Geometry: final body of the model. Coordinates: model frame, mm. A direction names the side the tool comes from. Coordinates: 2 decimals unless noted, no trailing zeros. Order: outer loops, then holes, each group sorted by start corner. A loop starts at its lowest first (then second) coordinate and runs counter-clockwise, first axis right, second up. Notation, with made-up numbers: (59.5, -27) - (67.5, -27) arc R20 ccw to (67.5, -18) - close; hole circle Ø10 at (83.25, -17). An arc over 180 degrees is marked (long way). Use a Markdown table: item, result. Add a question column.
```python
from build123d import *

# Parameters (mm, degrees)
SKETCH_1_R                   = 1.25
SKETCH_1_R_2                 = 1
EXTRUDE_1_DEPTH              = 5
SKETCH_3_W                   = 35
SKETCH_3_H                   = 7.5
EXTRUDE_2_DEPTH              = 12.5
SKETCH_5_R                   = 2.25
CUT_EXTRUDE_1_DEPTH          = 7.5
FILLET_2_R                   = 40
HOLE_WIZARD_M3_1_D           = 3.2
HOLE_WIZARD_M3_1_CBORE_D     = 6
HOLE_WIZARD_M3_1_CBORE_DEPTH = 3.4
CUT_EXTRUDE_2_DEPTH          = 48.681233206
FILLET_1_R                   = 2


with BuildPart() as part:
    # 草图1 → 凸台-拉伸1 (new body)
    # profile 1 of 2: a face of its own
    with BuildSketch(Plane.XY):
        with BuildLine():
            ThreePointArc((12.5, 18.708286934), (0, 22.5), (-12.5, 18.708286934))
            ThreePointArc((-12.5, 18.708286934), (-22.487606156, -0.746705683), (-11.231408892, -19.496293348))
            Line((-11.231408892, -19.496293348), (-5.24132415, -9.098270229))
            ThreePointArc((-5.24132415, -9.098270229), (-5.254336134, 9.090761892), (10.5, 0))
            ThreePointArc((10.5, 0), (9.090761892, -5.254336134), (5.24132415, -9.098270229))
            Line((5.24132415, -9.098270229), (11.231408892, -19.496293348))
            ThreePointArc((11.231408892, -19.496293348), (19.480204055, -11.259291717), (22.5, 0))
            ThreePointArc((22.5, 0), (19.843134833, 10.606601718), (12.5, 18.708286934))
        make_face()
        with Locations((-13.611805538, -13.611805538)):
            Circle(SKETCH_1_R, mode=Mode.SUBTRACT)
        with Locations((-10.25, -8)):
            Circle(SKETCH_1_R_2, mode=Mode.SUBTRACT)
        with Locations((10.25, -8)):
            Circle(SKETCH_1_R_2, mode=Mode.SUBTRACT)
        with Locations((13.611805538, -13.611805538)):
            Circle(SKETCH_1_R, mode=Mode.SUBTRACT)
        with Locations((-13.611805538, 13.611805538)):
            Circle(SKETCH_1_R, mode=Mode.SUBTRACT)
        with Locations((-10.25, 8)):
            Circle(SKETCH_1_R_2, mode=Mode.SUBTRACT)
        with Locations((10.25, 8)):
            Circle(SKETCH_1_R_2, mode=Mode.SUBTRACT)
        with Locations((13.611805538, 13.611805538)):
            Circle(SKETCH_1_R, mode=Mode.SUBTRACT)
    # profile 2 of 2: a face of its own
    with BuildSketch(Plane.XY):
        with BuildLine():
            Line((-12.5, 37.5), (-12.5, 18.708286934))
            ThreePointArc((-12.5, 18.708286934), (0, 22.5), (12.5, 18.708286934))
            Line((12.5, 18.708286934), (12.5, 37.5))
            Line((12.5, 37.5), (-12.5, 37.5))
        make_face()
    extrude(amount=EXTRUDE_1_DEPTH)

    # 草图3 → 凸台-拉伸2 (add, symmetric)
    with BuildSketch(Plane(origin=(0, 0, 0), x_dir=(0, 0, -1), z_dir=(1, 0, 0))):
        with Locations((-3.5, 33.75)):
            Rectangle(SKETCH_3_W, SKETCH_3_H)
    extrude(amount=EXTRUDE_2_DEPTH, both=True)

    # 草图5 → 切除-拉伸1 (cut, symmetric)
    with BuildSketch(Plane.XZ.offset(-30)):
        with Locations(Location((0, 3.5, 0), (0, 0, 270))):
            Circle(SKETCH_5_R)
    extrude(amount=CUT_EXTRUDE_1_DEPTH, both=True, mode=Mode.SUBTRACT)

    # 圆角2
    # the kernel refuses this fillet: 40 mm, written as the material it adds along each edge
    with BuildSketch(Plane(origin=(-12.5, 18.708286934, -38.008407454), x_dir=(-0.7015991579933682, -0.7125718360298817, 0), z_dir=(0, 0, 1))) as fillet_2_piece_1_section:
        with BuildLine():
            CenterArc((17.230478046, -39.169540108), FILLET_2_R, 101.695565513, 32.859880379)
            Line((-10.833488274, -10.666666667), (0, 0))
            ThreePointArc((0, 0), (4.561008895, -0.467133689), (9.122017789, 0))
        make_face()
    fillet_2_piece_1 = extrude(amount=43.008407454, mode=Mode.PRIVATE)
    fillet_2_piece_1 = split(fillet_2_piece_1, bisect_by=Plane(origin=(-12.133812824, 31.883513777, 0), z_dir=(0, 0, -1)), keep=Keep.TOP, mode=Mode.PRIVATE)
    fillet_2_piece_1 = split(fillet_2_piece_1, bisect_by=Plane(origin=(-12.133812824, 30, -7), z_dir=(0, 1, 0)), keep=Keep.TOP, mode=Mode.PRIVATE)
    fillet_2_piece_1 = split(fillet_2_piece_1, bisect_by=Plane(origin=(-12.133812824, 31.883513777, -14), z_dir=(0, 0, 1)), keep=Keep.TOP, mode=Mode.PRIVATE)
    add(fillet_2_piece_1)
    with BuildSketch(Plane(origin=(-12.5, 18.708286934, 0), x_dir=(-0.7015991579933694, -0.7125718360298806, 0), z_dir=(0, 0, 1))) as fillet_2_piece_2_section:
        with BuildLine():
            CenterArc((17.230478046, -39.169540108), FILLET_2_R, 101.695565513, 32.859880379)
            Line((-10.833488274, -10.666666667), (0, 0))
            ThreePointArc((0, 0), (4.561008895, -0.467133689), (9.122017789, 0))
        make_face()
    fillet_2_piece_2 = extrude(amount=5, mode=Mode.PRIVATE)
    fillet_2_piece_2 = split(fillet_2_piece_2, bisect_by=Plane(origin=(-13.82835822, 30, 2.5), z_dir=(0, -1, 0)), keep=Keep.TOP, mode=Mode.PRIVATE)
    add(fillet_2_piece_2)
    with BuildSketch(Plane(origin=(-12.5, 18.708286934, 0), x_dir=(-0.7015991579933694, -0.7125718360298806, 0), z_dir=(0, 0, 1))) as fillet_2_piece_3_section:
        with BuildLine():
            CenterArc((17.230478046, -39.169540108), FILLET_2_R, 101.695565513, 32.859880379)
            Line((-10.833488274, -10.666666667), (0, 0))
            ThreePointArc((0, 0), (4.561008895, -0.467133689), (9.122017789, 0))
        make_face()
    fillet_2_piece_3 = extrude(amount=5, mode=Mode.PRIVATE)
    fillet_2_piece_3 = split(fillet_2_piece_3, bisect_by=Plane(origin=(-12.133812824, 30, 2.5), z_dir=(0, 1, 0)), keep=Keep.TOP, mode=Mode.PRIVATE)
    add(fillet_2_piece_3)
    with BuildSketch(Plane(origin=(-12.5, 18.708286934, 0), x_dir=(-0.7015991579933694, -0.7125718360298806, 0), z_dir=(0, 0, 1))) as fillet_2_piece_4_section:
        with BuildLine():
            CenterArc((17.230478046, -39.169540108), FILLET_2_R, 101.695565513, 32.859880379)
            Line((-10.833488274, -10.666666667), (0, 0))
            ThreePointArc((0, 0), (4.561008895, -0.467133689), (9.122017789, 0))
        make_face()
    fillet_2_piece_4 = extrude(amount=43.008407454, mode=Mode.PRIVATE)
    fillet_2_piece_4 = split(fillet_2_piece_4, bisect_by=Plane(origin=(-12.133812824, 31.883513777, 5), z_dir=(0, 0, 1)), keep=Keep.TOP, mode=Mode.PRIVATE)
    fillet_2_piece_4 = split(fillet_2_piece_4, bisect_by=Plane(origin=(-12.133812824, 30, 13), z_dir=(0, 1, 0)), keep=Keep.TOP, mode=Mode.PRIVATE)
    fillet_2_piece_4 = split(fillet_2_piece_4, bisect_by=Plane(origin=(-12.133812824, 31.883513777, 21), z_dir=(0, 0, -1)), keep=Keep.TOP, mode=Mode.PRIVATE)
    add(fillet_2_piece_4)
    with BuildSketch(Plane(origin=(12.5, 18.708286934, -38.008407454), x_dir=(0.7015991579933666, -0.7125718360298834, 0), z_dir=(0, 0, 1))) as fillet_2_piece_5_section:
        with BuildLine():
            CenterArc((17.230478046, 39.169540108), FILLET_2_R, 225.444554108, 32.859880379)
            Line((-10.833488274, 10.666666667), (0, 0))
            ThreePointArc((0, 0), (4.561008895, 0.467133689), (9.122017789, 0))
        make_face()
    fillet_2_piece_5 = extrude(amount=43.008407454, mode=Mode.PRIVATE)
    fillet_2_piece_5 = split(fillet_2_piece_5, bisect_by=Plane(origin=(12.133812824, 31.883513777, 0), z_dir=(0, 0, -1)), keep=Keep.TOP, mode=Mode.PRIVATE)
    fillet_2_piece_5 = split(fillet_2_piece_5, bisect_by=Plane(origin=(12.133812824, 30, -7), z_dir=(0, 1, 0)), keep=Keep.TOP, mode=Mode.PRIVATE)
    fillet_2_piece_5 = split(fillet_2_piece_5, bisect_by=Plane(origin=(12.133812824, 31.883513777, -14), z_dir=(0, 0, 1)), keep=Keep.TOP, mode=Mode.PRIVATE)
    add(fillet_2_piece_5)
    with BuildSketch(Plane(origin=(12.5, 18.708286934, 0), x_dir=(0.7015991579933667, -0.7125718360298833, 0), z_dir=(0, 0, 1))) as fillet_2_piece_6_section:
        with BuildLine():
            CenterArc((17.230478046, 39.169540108), FILLET_2_R, 225.444554108, 32.859880379)
            Line((-10.833488274, 10.666666667), (0, 0))
            ThreePointArc((0, 0), (4.561008895, 0.467133689), (9.122017789, 0))
        make_face()
    fillet_2_piece_6 = extrude(amount=5, mode=Mode.PRIVATE)
    fillet_2_piece_6 = split(fillet_2_piece_6, bisect_by=Plane(origin=(13.82835822, 30, 2.5), z_dir=(0, -1, 0)), keep=Keep.TOP, mode=Mode.PRIVATE)
    add(fillet_2_piece_6)
    with BuildSketch(Plane(origin=(12.5, 18.708286934, 0), x_dir=(0.7015991579933667, -0.7125718360298833, 0), z_dir=(0, 0, 1))) as fillet_2_piece_7_section:
        with BuildLine():
            CenterArc((17.230478046, 39.169540108), FILLET_2_R, 225.444554108, 32.859880379)
            Line((-10.833488274, 10.666666667), (0, 0))
            ThreePointArc((0, 0), (4.561008895, 0.467133689), (9.122017789, 0))
        make_face()
    fillet_2_piece_7 = extrude(amount=5, mode=Mode.PRIVATE)
    fillet_2_piece_7 = split(fillet_2_piece_7, bisect_by=Plane(origin=(12.133812824, 30, 2.5), z_dir=(0, 1, 0)), keep=Keep.TOP, mode=Mode.PRIVATE)
    add(fillet_2_piece_7)
    with BuildSketch(Plane(origin=(12.5, 18.708286934, 0), x_dir=(0.7015991579933667, -0.7125718360298833, 0), z_dir=(0, 0, 1))) as fillet_2_piece_8_section:
        with BuildLine():
            CenterArc((17.230478046, 39.169540108), FILLET_2_R, 225.444554108, 32.859880379)
            Line((-10.833488274, 10.666666667), (0, 0))
            ThreePointArc((0, 0), (4.561008895, 0.467133689), (9.122017789, 0))
        make_face()
    fillet_2_piece_8 = extrude(amount=43.008407454, mode=Mode.PRIVATE)
    fillet_2_piece_8 = split(fillet_2_piece_8, bisect_by=Plane(origin=(12.133812824, 31.883513777, 5), z_dir=(0, 0, 1)), keep=Keep.TOP, mode=Mode.PRIVATE)
    fillet_2_piece_8 = split(fillet_2_piece_8, bisect_by=Plane(origin=(12.133812824, 30, 13), z_dir=(0, 1, 0)), keep=Keep.TOP, mode=Mode.PRIVATE)
    fillet_2_piece_8 = split(fillet_2_piece_8, bisect_by=Plane(origin=(12.133812824, 31.883513777, 21), z_dir=(0, 0, -1)), keep=Keep.TOP, mode=Mode.PRIVATE)
    add(fillet_2_piece_8)

    # M3 六角圆柱头螺钉的柱形沉头孔1 (through all)
    with Locations(Plane(origin=(0, 30, 0), x_dir=(-1, 0, 0), z_dir=(0, -1, 0))):
        with Locations((8.838834765, -12.338834765), (-8.838834765, -12.338834765), (-8.838834765, 5.338834765), (8.838834765, 5.338834765)):
            CounterBoreHole(HOLE_WIZARD_M3_1_D / 2, HOLE_WIZARD_M3_1_CBORE_D / 2, HOLE_WIZARD_M3_1_CBORE_DEPTH)

    # 草图9 → 切除-拉伸2 (cut, through all)
    with BuildSketch(Plane.XY.offset(5)):
        Polygon((-4, 30), (-8.5, 18.164414003), (-8.5, 6.164414003), (8.5, 6.164414003), (8.5, 18.164414003), (4, 30), align=None)
    extrude(amount=-CUT_EXTRUDE_2_DEPTH, mode=Mode.SUBTRACT)

    # 圆角1
    fillet_1_edges = [part.edges().sort_by_distance(p)[0] for p in [
        (8.5, 6.164414003, 2.5),
        (-8.5, 6.164414003, 2.5),
        (-8.5, 18.164414003, 2.5),
        (4, 30, 2.5),
        (8.5, 18.164414003, 2.5),
        (-4, 30, 2.5),
        (11.231408892, -19.496293348, 2.5),
        (5.24132415, -9.098270229, 2.5),
        (-5.24132415, -9.098270229, 2.5),
        (-11.231408892, -19.496293348, 2.5),
        (-12.5, 35.705824958, 21),
        (12.5, 35.705824958, 21),
        (-12.5, 35.705824958, -14),
        (12.5, 35.705824958, -14),
        (-12.547959259, 31.953477145, -14),
        (-12.547959259, 31.953477145, 21),
        (12.547959259, 31.953477145, -14),
        (12.547959259, 31.953477145, 21),
    ]]
    fillet(fillet_1_edges, radius=FILLET_1_R)


solid = part.part
```
1) Section C-C (y = 21.5). Return loops of the section in (x, z).
2) Ray query, line 1 along Y through (x, z) = (3.5, 6); line 2 along Z through (x, y) = (8, 21); line 3 along X through (y, z) = (16, 0.5). Return the intervals inside material, ascending.
3) Pin query (flat end, axial travel): pin 1 (10 mm diameter, centred on y = 15.5, z = -6, fed in from +X); pin 2 (2.5 mm diameter, centred on x = 10.25, y = 8, fed in from +Z); pin 3 (6 mm diameter, centred on x = 0, z = 3.5, fed in from -Y); pin 4 (2.5 mm diameter, centred on x = -10.25, y = -8, fed in from -Z). Return the tip coordinate at first contact, or that it passes through.
4) Section A-A (z = -4.5). Return loops of the section in (x, y), then the cut area to 3 significant figures.
5) Draft query along Z for faces 6 (the face through (-11.93, 35.73, 20.4)), 7 (the face through (8, 33.4, 14)), 8 (the face through (12.5, 36, 4)). Return one class per face: pulls with the +Z half, pulls with the -Z half, needs draft (parallel to the pull), parting line crosses it, or undercut.
6) Section D-D (z = 3.5). Give the number of separate pieces and of enclosed holes in the cut face, then the cut area to 3 significant figures.
7) Set-up query: faces 1 (the face through (14, 5, 0)), 2 (the face through (-10, 33.4, 14)), 3 (the face through (-3.77, 29.637, 2.465)), 4 (the face through (11.93, 35.73, -13.4)), 5 (the face through (-6.403, 23.681, 2.535)). Return all of +Z, -Z, +X, -X, +Y, -Y with unobstructed straight access to the full face (end or side cutting, diameter ignored); none if empty.
8) Section B-B (y = 8). Return loops of the section in (x, z).
Values follow:
| question | item | result |
|---|---|---|
| 1 | outline | (-14.47, 0) - (-7.23, 0) - (-7.23, 5) - (-14.47, 5) - close; (7.23, 0) - (14.47, 0) - (14.47, 5) - (7.23, 5) - close |
| 2 | line 1 | y = 30 to 37.5 |
| 2 | line 2 | z = 0 to 5 |
| 2 | line 3 | x = -16.73 to -8.5, 8.5 to 16.73 |
| 3 | pin 1 | passes through |
| 3 | pin 2 | stops at z = 5 |
| 3 | pin 3 | stops at y = 29.96 |
| 3 | pin 4 | stops at z = 0 |
| 4 | outline | (-12.69, 30) - (-11.72, 30) - (-11.72, 33.4) - (-10.2, 33.4) - (-10.2, 37.5) - (-12.5, 37.5) - (-12.5, 33.91) arc R40 cw to start; (-7.48, 33.4) - (-5.96, 33.4) - (-5.96, 30) - (5.96, 30) - (5.96, 33.4) - (7.48, 33.4) - (7.48, 37.5) - (-7.48, 37.5) - close; (10.2, 33.4) - (11.72, 33.4) - (11.72, 30) - (12.69, 30) arc R40 cw to (12.5, 33.91) - (12.5, 37.5) - (10.2, 37.5) - close |
| 4 | area | 126 mm² |
| 5 | face 6 | pulls with the +Z half |
| 5 | face 7 | undercut |
| 5 | face 8 | needs draft |
| 6 | separate pieces | 2 |
| 6 | enclosed holes | 8 |
| 6 | area | 1,120 mm² |
| 7 | face 1 | -Z, +X, -X, -Y |
| 7 | face 2 | -Y |
| 7 | face 3 | +Z, -Z, -Y |
| 7 | face 4 | -Z, +X, +Y |
| 7 | face 5 | +Z, -Z |
| 8 | outline | (-21.03, 0) - (-11.25, 0) - (-11.25, 5) - (-21.03, 5) - close; (-9.25, 0) - (-8.5, 0) - (-8.5, 5) - (-9.25, 5) - close; (8.5, 0) - (9.25, 0) - (9.25, 5) - (8.5, 5) - close; (11.25, 0) - (21.03, 0) - (21.03, 5) - (11.25, 5) - close |
